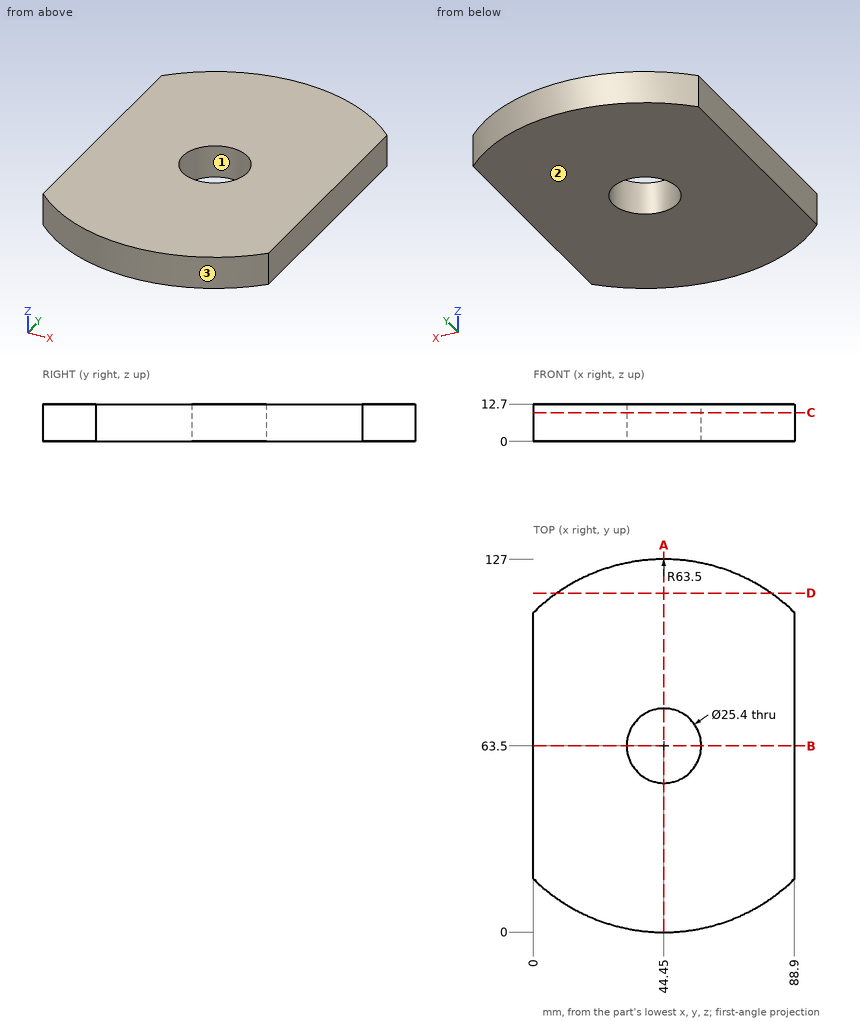
For this review, use the dimensioned drawing (mm, ordinates from the lowest corner) and the shaded views. Round coordinates to 2 decimals unless told otherwise and drop trailing zeros. Order: outer loops, then holes, each group sorted by start corner. A loop starts at its lowest first (then second) coordinate and runs counter-clockwise, first axis right, second up. Notation, with made-up numbers: M 72.5,46 L 119.5,46 A19 cw 119.5,70 Z; hole C 15.5,-29.5 d4. An arc over 180 degrees is marked long. Use a Markdown table: item, result. Add a question column.
Item 1: Add section A-A, the plane x = 44.45. Give the boundary of the cut face in (y, z), then the cut area to 3 significant figures.
Item 2: Mouldability with a two-part tool opening along X and no side actions: class the marked faces 1, 2 and 3 as released by +X, released by -X, zero draft, split by the parting line, or undercut.
Item 3: Insertion check: pin 1 (6 mm diameter, centred on y = 13.5, z = 5, fed in from -X); pin 2 (2 mm diameter, centred on x = 24.5, z = 6, fed in from -Y); pin 3 (4 mm diameter, centred on x = 39.5, z = 9, fed in from -Y). Each pin has a flat end and moves straight along its axis. Give the tip position at first contact, or say it passes through.
Item 4: Add section B-B, the plane y = 63.5. Give the boundary of the cut face in (x, z).
Item 5: To check wall thickness, follow line 1 along Y through (x, z) = (34, 0.5); line 2 along Y through (x, z) = (36, 1.5); line 3 along X through (y, z) = (7, 8.5). State the ranges of each line that lie inside material, in increasing order.
Item 6: Add section D-D, the plane y = 115.5. Give the boundary of the cut face in (x, z).
Item 7: Add section C-C, the plane z = 9.75. Give the boundary of the cut face in (x, y), then the cut area to 3 significant figures.
Geometry results:
| question | item | result |
|---|---|---|
| 1 | outline | M 0,0 L 50.8,0 L 50.8,12.7 L 0,12.7 Z; M 76.2,0 L 127,0 L 127,12.7 L 76.2,12.7 Z |
| 1 | area | 1,290 mm² |
| 2 | face 1 | undercut |
| 2 | face 2 | zero draft |
| 2 | face 3 | split by the parting line |
| 3 | pin 1 | stops at x = 1.75 |
| 3 | pin 2 | stops at y = 2.89 |
| 3 | pin 3 | stops at y = 0.07 |
| 4 | outline | M 0,0 L 31.75,0 L 31.75,12.7 L 0,12.7 Z; M 57.15,0 L 88.9,0 L 88.9,12.7 L 57.15,12.7 Z |
| 5 | line 1 | y = 0.87 to 56.28, 70.72 to 126.13 |
| 5 | line 2 | y = 0.56 to 54.02, 72.98 to 126.44 |
| 5 | line 3 | x = 15.47 to 73.43 |
| 6 | outline | M 8,0 L 80.9,0 L 80.9,12.7 L 8,12.7 Z |
| 7 | outline | M 0,18.15 A63.5 ccw 88.9,18.15 L 88.9,108.85 A63.5 ccw 0,108.85 Z; hole C 44.45,63.5 d25.4 |
| 7 | area | 9,780 mm² |
